```python
from build123d import *

# Parameters (mm, degrees)
SKETCH1_W           = 4.6228
SKETCH1_H           = 12.5349
BOSS_EXTRUDE1_DEPTH = 2.38125
BOSS_EXTRUDE2_DEPTH = 6.35
SKETCH3_W           = 0.791761441
SKETCH3_H           = 4.7625
BOSS_EXTRUDE3_DEPTH = 0.79375
SKETCH4_W           = 0.791761441
SKETCH4_H           = 4.7625
BOSS_EXTRUDE4_DEPTH = 0.79375
FILLET1_R           = 1.27
SHELL1_START        = -1.8542
SHELL1_OUTLINE_W    = 5.334
SHELL1_OUTLINE_H    = 8.9662
SHELL1_DEPTH        = 6.477
SHELL1_START_2      = 0.508
SHELL1_2_OUTLINE_W  = 1.36525
SHELL1_2_OUTLINE_H  = 1.27635
SHELL1_2_DEPTH      = 4.1148


# Read off the part's stored shape, not the designer's step: Shell1
with BuildPart() as part:
    # Sketch1 → Boss-Extrude1 (new body)
    with BuildSketch(Plane(origin=(0, 0, 0), x_dir=(1, 0, 0), z_dir=(0, 1, 0))):
        with Locations((2.3114, 6.26745)):
            Rectangle(SKETCH1_W, SKETCH1_H)
    extrude(amount=BOSS_EXTRUDE1_DEPTH)

    # Sketch2 → Boss-Extrude2 (add)
    with BuildSketch(Plane(origin=(0, 0, 0), x_dir=(-1, 0, 0), z_dir=(0, -1, 0))):
        Polygon((-4.6228, 6.26745), (-4.6228, 11.25855), (2.3622, 11.25855), (2.3622, 1.27635), (-4.6228, 1.27635), align=None)
    extrude(amount=-BOSS_EXTRUDE2_DEPTH)

    # Sketch3 → Boss-Extrude3 (add)
    with BuildSketch(Plane.XY.offset(-1.27635)):
        with Locations((-2.758080721, 2.38125)):
            Rectangle(SKETCH3_W, SKETCH3_H)
    extrude(amount=-BOSS_EXTRUDE3_DEPTH)

    # Sketch4 → Boss-Extrude4 (add)
    with BuildSketch(Plane(origin=(0, 0, -11.25855), x_dir=(-1, 0, 0), z_dir=(0, 0, -1))):
        with Locations((2.758080721, 2.38125)):
            Rectangle(SKETCH4_W, SKETCH4_H)
    extrude(amount=-BOSS_EXTRUDE4_DEPTH)

    # Fillet1
    # the kernel refuses this fillet: 1.27 mm, written as the material it takes off along each edge
    with BuildSketch(Plane(origin=(-3.153961441, 4.7625, 1.664937857), x_dir=(1, 0, 0), z_dir=(0, 0, -1))) as fillet1_piece_1:
        with BuildLine():
            CenterArc((1.27, 1.176515143), FILLET1_R, 180, 67.878878404)
            Line((0, 1.176515143), (-0.0254, 1.176515143))
            Line((-0.0254, 1.176515143), (-0.0254, 0))
            Line((-0.0254, 0), (0, -0.0254))
            ThreePointArc((0, -0.0254), (0.395880721, -0.0254), (0.78219667, -0.023530303))
            Line((0.78219667, -0.023530303), (0.791761441, 0))
        make_face()
    extrude(amount=6.676325713, mode=Mode.SUBTRACT)
    with BuildSketch(Plane(origin=(-3.153961441, 4.7625, -14.199837857), x_dir=(0, -1, 0), z_dir=(0, 0, 1))) as fillet1_piece_2:
        with BuildLine():
            CenterArc((1.176515143, 1.27), FILLET1_R, 202.121121596, 67.878878404)
            Line((0, 0.791761441), (-0.023530303, 0.78219667))
            ThreePointArc((-0.023530303, 0.78219667), (-0.0254, 0.395880721), (-0.0254, 0))
            Line((-0.0254, 0), (0, -0.0254))
            Line((0, -0.0254), (1.176515143, -0.0254))
            Line((1.176515143, -0.0254), (1.176515143, 0))
        make_face()
    extrude(amount=6.676325713, mode=Mode.SUBTRACT)

    # Shell1 outline → Shell1 (cut)
    with BuildSketch(Plane.YZ.offset(SHELL1_START)):
        with Locations((3.175, -6.26745)):
            Rectangle(SHELL1_OUTLINE_W, SHELL1_OUTLINE_H)
    extrude(amount=SHELL1_DEPTH, mode=Mode.SUBTRACT)

    # Shell1 2 outline → Shell1 2 (cut)
    with BuildSketch(Plane.YZ.offset(SHELL1_START_2)):
        with Locations((1.190625, -11.388725)):
            Rectangle(SHELL1_2_OUTLINE_W, SHELL1_2_OUTLINE_H)
        with Locations((1.190625, -1.146175)):
            Rectangle(SHELL1_2_OUTLINE_W, SHELL1_2_OUTLINE_H)
    extrude(amount=SHELL1_2_DEPTH, mode=Mode.SUBTRACT)


solid = part.part
```
Build history of the part. All positions in model axes, mm. A direction names the side the tool comes from. Coordinates: 2 decimals unless noted, no trailing zeros. Write each loop counter-clockwise with the first axis right and the second up, starting at its lowest first coordinate (ties: lowest second). Pieces come first, ordered by that corner, then holes.
1. Band-saw the part on B-B, the plane z = -6. Give the cut face in (x, y).
Answer block:
outline: (-2.36, 0) - (4.62, 0) - (4.62, 0.51) - (-1.85, 0.51) - (-1.85, 5.84) - (4.62, 5.84) - (4.62, 6.35) - (-2.36, 6.35) - close
2. Band-saw the part on A-A, the plane x = 3.5. Give the cut face in (y, z).
Answer block:
outline: (0, -12.53) - (2.38, -12.53) - (2.38, -11.26) - (6.35, -11.26) - (6.35, -1.28) - (2.38, -1.28) - (2.38, 0) - (0, 0) - close; hole (0.51, -12.03) - (1.87, -12.03) - (1.87, -10.75) - (5.84, -10.75) - (5.84, -1.78) - (1.87, -1.78) - (1.87, -0.51) - (0.51, -0.51) - close
3. Drill centre lines: probe 1 along Z at (x, y) = (1.5, 4); probe 2 along Z at (x, y) = (-2.5, 3.5); probe 3 along Y at (x, z) = (2.5, -9.75). Where is each one in solid material? Low to high.
Answer block:
probe 1: z = -11.26 to -10.75, -1.78 to -1.28
probe 2: z = -11.26 to -10.46, -2.07 to -1.28
probe 3: y = 0 to 0.51, 5.84 to 6.35
4. Band-saw the part on D-D, the plane x = -2.5. Give the cut face in (y, z).
Answer block:
outline: (0, -11.26) - (4.7, -11.26) - (4.7, -10.46) - (0, -10.46) - close; (0, -2.07) - (4.7, -2.07) - (4.7, -1.28) - (0, -1.28) - close
5. 3-axis set-ups, long thin cutter, end or side, ignore diameter. For faces 4 (the flat face through (0, 1, -12)), 5 (the flat face through (0.508, 1, -1)), 6 (the flat face through (0, 1, -1)), 7 (the flat face through (4.623, 0.3, -6.2)): which of +Z, -Z, +X, -X, +Y, -Y reach the whole face in a straight line?
Answer block:
face 4: -Z, -X, +Y, -Y
face 5: +X
face 6: +Z, -X, +Y, -Y
face 7: +Z, -Z, +X, +Y, -Y
6. Pull direction Z, two halves, no side cores. Call faces 1 (the flat face through (1, 0.508, -6)), 2 (the flat face through (2, 1, 0)), 3 (the flat face through (2, 2.381, -12)): released by +Z, released by -Z, zero draft, split by the parting line, or undercut.
Answer block:
face 1: undercut
face 2: released by +Z
face 3: zero draft
7. Band-saw the part on C-C, the plane y = 5.25. Give the cut face in (x, z), and give its area (3 significant figures).
Answer block:
outline: (-2.36, -11.26) - (4.62, -11.26) - (4.62, -10.75) - (-1.85, -10.75) - (-1.85, -1.78) - (4.62, -1.78) - (4.62, -1.28) - (-2.36, -1.28) - close
area: 11.7 mm2
8. Drop flat-ended pins along their axis: pin 1 (1.4 mm diameter, centred on x = 2.5, z = -0.5, fed in from +Y); pin 2 (2.5 mm diameter, centred on x = 1.5, y = 4.5, fed in from -Z); pin 3 (0.6 mm diameter, centred on y = 1, z = -1, fed in from +X). Give the stop position or say it passes through.
Answer block:
pin 1: stops at y = 2.38
pin 2: stops at z = -11.26
pin 3: stops at x = 0.51
